Build history of the part. All positions in model axes, mm. Give positions to 0.01 mm unless a question says otherwise; leave off trailing zeros. Write each loop counter-clockwise with the first axis right and the second up, starting at its lowest first coordinate (ties: lowest second). Pieces come first, ordered by that corner, then holes.
from build123d import *

# Parameters (mm, degrees)
SKETCH1_W           = 465
SKETCH1_H           = 20
BOSS_EXTRUDE1_DEPTH = 30
FILLET1_R           = 2
SKETCH3_R           = 4
CUT_EXTRUDE2_DEPTH  = 236.279089594
SKETCH5_R           = 5
CUT_EXTRUDE4_DEPTH  = 236.279089594
SKETCH8_R           = 4
CUT_EXTRUDE5_DEPTH  = 236.279089594


with BuildPart() as part:
    # Sketch1 → Boss-Extrude1 (new body)
    with BuildSketch(Plane.XY):
        with Locations((0, 10)):
            Rectangle(SKETCH1_W, SKETCH1_H)
    extrude(amount=BOSS_EXTRUDE1_DEPTH)

    # Fillet1
    fillet1_edges = [part.edges().sort_by_distance(p)[0] for p in [
        (232.5, 10, 30),
        (0, 20, 30),
        (0, 20, 0),
        (232.5, 10, 0),
        (0, 0, 0),
        (-232.5, 10, 0),
        (-232.5, 20, 15),
        (232.5, 20, 15),
        (232.5, 0, 15),
        (-232.5, 0, 15),
        (0, 0, 30),
    ]]
    fillet(fillet1_edges, radius=FILLET1_R)

    # Sketch3 → Cut-Extrude2 (cut, through all)
    with BuildSketch(Plane(origin=(0, 20, 0), x_dir=(1, 0, 0), z_dir=(0, 1, 0))):
        with Locations(Location((-216.9, -15, 0), (0, 0, 270))):
            Circle(SKETCH3_R)
    extrude(amount=-CUT_EXTRUDE2_DEPTH, mode=Mode.SUBTRACT)

    # Sketch5 → Cut-Extrude4 (cut, through all)
    with BuildSketch(Plane.XY.offset(30)):
        with Locations((212.5, 10)):
            Circle(SKETCH5_R)
    extrude(amount=-CUT_EXTRUDE4_DEPTH, mode=Mode.SUBTRACT)

    # Sketch8 → Cut-Extrude5 (cut, through all)
    with BuildSketch(Plane(origin=(0, 20, 0), x_dir=(1, 0, 0), z_dir=(0, 1, 0))):
        with Locations(Location((222.5, -15, 0), (0, 0, 270))):
            Circle(SKETCH8_R)
    extrude(amount=-CUT_EXTRUDE5_DEPTH, mode=Mode.SUBTRACT)


solid = part.part
(1) Probe line 1 (X direction, y = 8.5, z = 15); line 2 (X direction, y = 17.5, z = 18.5); line 3 (X direction, y = 9.25, z = 23.25). List the from-to ranges inside material, lowest first.
(2) Saw through at A-A, the plane z = 15. List the corners of the cut face in (x, y), plus the area to 3 significant figures.
(3) Saw through at B-B, the plane x = 212.5. List the corners of the cut face in (y, z).
(4) Saw through at C-C, the plane x = -216.9. List the corners of the cut face in (y, z), plus the area to 3 significant figures.
(5) Mould opens along Z. For faces 1 (the face through (-220.805, 10.14, 14.133)), 2 (the face through (225.873, 10.14, 17.15)), 3 (the face through (-4, 10, 30)), 4 (the face through (-232.5, 10, 16)) say: +Z half, -Z half, draft (parallel to the pull), parting line (faces both ways), or undercut.
Computed values:
1. line 1: x = -232.5 to -220.9, -212.9 to 207.73, 217.27 to 218.5, 226.5 to 232.5
1. line 2: x = -232.5 to -218.84, -214.96 to 220.56, 224.44 to 232.5
1. line 3: x = -232.5 to 207.56, 217.44 to 232.5
2. outline: (-232.5, 2) arc R2 ccw to (-230.5, 0) - (-220.9, 0) - (-220.9, 20) - (-230.5, 20) arc R2 ccw to (-232.5, 18) - close; (-212.9, 0) - (218.5, 0) - (218.5, 20) - (-212.9, 20) - close; (226.5, 0) - (230.5, 0) arc R2 ccw to (232.5, 2) - (232.5, 18) arc R2 ccw to (230.5, 20) - (226.5, 20) - close; hole circle Ø10 at (212.5, 10)
2. area: 8,900 mm2
3. outline: (0, 2) arc R2 ccw to (2, 0) - (5, 0) - (5, 30) - (2, 30) arc R2 ccw to (0, 28) - close; (15, 0) - (18, 0) arc R2 ccw to (20, 2) - (20, 28) arc R2 ccw to (18, 30) - (15, 30) - close
4. outline: (0, 2) arc R2 ccw to (2, 0) - (18, 0) arc R2 ccw to (20, 2) - (20, 11) - (0, 11) - close; (0, 19) - (20, 19) - (20, 28) arc R2 ccw to (18, 30) - (2, 30) arc R2 ccw to (0, 28) - close
4. area: 437 mm2
5. face 1: undercut
5. face 2: undercut
5. face 3: +Z half
5. face 4: draft
